Build history of the part. All positions in model axes, mm. A direction names the side the tool comes from. Give positions to 0.01 mm unless a question says otherwise; leave off trailing zeros. Loops run counter-clockwise (first coordinate to the right, second up) from the corner with the lowest first, then second, coordinate; pieces in that order, holes last. Notation, with made-up numbers: (-22.75, 21.5) - (19.25, 21.5) arc R24 cw to (19.25, 56.5) - close; hole circle Ø9 at (-1, 71.25). An arc over 180 degrees is marked (long way). Return JSON: item names as keys, results as strings. Group by question number.
1) Slice it at A-A (x = 5). List the corners of the cut face in (y, z).
2) Slice it at B-B (z = -0.5). List the corners of the cut face in (x, y), and give its area (3 significant figures).
3) Slice it at C-C (y = -4.25). List the corners of the cut face in (x, z) (3 decimals), and give its area (3 significant figures).
4) Slice it at D-D (x = 43). List the corners of the cut face in (y, z).
5) Drill centre lines: probe 1 along X at (y, z) = (-0.75, -11); probe 2 along Z at (x, y) = (-4, -0.75); probe 3 along X at (y, z) = (-5, 0). Where is each one in solid material? Low to high. Write a range as from..to.
6) 3-axis set-ups, long thin cutter, end or side, ignore diameter. For faces 4 (the face through (54.54, -4.93, 18.38)), 5 (the face through (9.932, -4.93, -27.535)), 6 (the face through (-0.99, -4.93, -3.82)): which of +Z, -Z, +X, -X, +Y, -Y reach the whole face in a straight line?
7) Drop flat-ended pins along their axis: pin 1 (2 mm diameter, centred on x = -50.5, z = 22, fed in from +Y); pin 2 (3 mm diameter, centred on x = 27, z = -22.5, fed in from -Y); pin 3 (3 mm diameter, centred on y = -6, z = -16, fed in from -X); pin 4 (2 mm diameter, centred on y = -3, z = -14.5, fed in from -X). Give the stop position or say it passes through.
8) Mould opens along Z. For faces 1 (the face through (-54, -5, 21)), 2 (the face through (32.959, -5.07, 28.146)), 3 (the face through (-54.54, -4.93, -18.38)) say: released by +Z, released by -Z, zero draft, split by the parting line, or undercut.
```python
from build123d import *

# Parameters (mm, degrees)
F1_DEPTH = 10
F2_R     = 5
F3_R     = 5


with BuildPart() as f1:
    # F0 (on Front) → F1 (new body)
    with BuildSketch(Plane.XZ):
        Polygon((-75, 0), (-34, -36.828427), (33, 30.171573), (65, -1), (30, -30), (2.828427, -2.828427), (-11.313708, -16.970563), (35, -40), (75, 0), (34, 36.828427), (-33, -30.171573), (-65, 1), (-30, 30), (-2.828427, 2.828427), (11.313708, 16.970563), (-35, 40), align=None)
    extrude(amount=F1_DEPTH)

    # F2
    f2_edges = [f1.edges().sort_by_distance(p)[0] for p in [
        (-30, -5, 30),
        (-65, -5, 1),
        (-33, -5, -30.171573),
        (33, -5, 30.171573),
        (65, -5, -1),
        (30, -5, -30),
    ]]
    fillet(f2_edges, radius=F2_R)

    # F3
    f3_edges = [f1.edges().sort_by_distance(p)[0] for p in [
        (-35, -5, 40),
        (-75, -5, 0),
        (-34, -5, -36.828427),
        (35, -5, -40),
        (75, -5, 0),
        (34, -5, 36.828427),
    ]]
    fillet(f3_edges, radius=F3_R)


solid = f1.part
```
Results:
{
 "1": {"outline": "(-10, -25.08) - (0, -25.08) - (0, -5) - (-10, -5) - close; (-10, 2.17) - (0, 2.17) - (0, 7.83) - (-10, 7.83) - close; (-10, 10.66) - (0, 10.66) - (0, 20.11) - (-10, 20.11) - close"},
 "2": {"outline": "(-72.69, -10) - (-62.38, -10) - (-62.38, 0) - (-72.69, 0) - close; (-3.33, -10) - (2.33, -10) - (2.33, 0) - (-3.33, 0) - close; (62.52, -10) - (72.73, -10) - (72.73, 0) - (62.52, 0) - close", "area": "262 mm2"},
 "3": {"outline": "(-71.27, 3.73) arc R5 ccw to (-71.076, -3.525) - (-37.526, -33.661) arc R5 ccw to (-30.649, -33.477) - (29.511, 26.682) arc R5 cw to (36.535, 26.728) - (61.015, 2.882) arc R5 cw to (60.716, -4.55) - (33.506, -27.095) arc R5 cw to (26.78, -26.78) - (2.828, -2.828) - (-11.314, -16.971) - (31.781, -38.399) arc R5 ccw to (37.542, -37.458) - (71.27, -3.73) arc R5 ccw to (71.076, 3.525) - (37.526, 33.661) arc R5 ccw to (30.649, 33.477) - (-29.511, -26.682) arc R5 cw to (-36.535, -26.728) - (-61.015, -2.882) arc R5 cw to (-60.716, 4.55) - (-33.506, 27.095) arc R5 cw to (-26.78, 26.78) - (-2.828, 2.828) - (11.314, 16.971) - (-31.781, 38.399) arc R5 ccw to (-37.542, 37.458) - close", "area": "3,010 mm2"},
 "4": {"outline": "(-10, -32) - (0, -32) - (0, -19.23) - (-10, -19.23) - close; (-10, 20.43) - (0, 20.43) - (0, 28.74) - (-10, 28.74) - close"},
 "5": {"probe 1": "-62.75..-52.68, -13.83..-8.17, -5.34..11, 52.93..64", "probe 2": "-20.61..-9.66, -6.83..-1.17, 4..24.59", "probe 3": "-72.73..-62.48, -2.83..2.83, 62.48..72.73"},
 "6": {"face 4": "+Z, +X, +Y, -Y", "face 5": "-Z, +Y, -Y", "face 6": "+Y, -Y"},
 "7": {"pin 1": "y = 0", "pin 2": "through", "pin 3": "x = -58.86", "pin 4": "x = -59.97"},
 "8": {"face 1": "released by +Z", "face 2": "undercut", "face 3": "released by -Z"}
}
